```python
from build123d import *

# Parameters (mm, degrees)
F1_DEPTH = 12.7


with BuildPart() as f1:
    # F0 (on Right) → F1 (new body)
    with BuildSketch(Plane.YZ):
        with BuildLine():
            Line((-18.77171, -42.24451), (-18.77171, 60.838442))
            Line((-18.77171, 60.838442), (-29.627644, 60.838442))
            Line((-29.627644, 60.838442), (-29.627644, -38.221922))
            ThreePointArc((-29.627644, -38.221922), (-48.0446, -53.631362), (-69.885053, -43.64989))
            ThreePointArc((-69.885053, -43.64989), (-45.128132, -60.419661), (-19.449341, -45.098757))
            ThreePointArc((-19.449341, -45.098757), (-18.94344, -43.711302), (-18.77171, -42.24451))
        make_face()
    extrude(amount=F1_DEPTH)


solid = f1.part
```
For this review, take the finished solid that the model builds, in its own axes (mm). A direction names the side the tool comes from. Give positions to 0.01 mm unless a question says otherwise; leave off trailing zeros. Order: outer loops, then holes, each group sorted by start corner. A loop starts at its lowest first (then second) coordinate and runs counter-clockwise, first axis right, second up.
1) For faces 1 (the face through (12.7, -29, -8)), 2 (the face through (6, -29.628, 12)), list the 3-axis set-ups (+Z, -Z, +X, -X, +Y, -Y) from which the entire face can be reached by the end or side of a thin tool; tool diameter is ignored.
2) Take a section at A-A (x = 9.5). Give the boundary of the cut face in (y, z).
3) Wall thickness on line 1 (Y direction, x = 7.5, z = 51.5); line 2 (Y direction, x = 1.5, z = -51.5); line 3 (Z direction, x = 3.25, y = -40): over which ranges is each line inside the solid? List them lowest first.
4) Take a section at B-B (z = 19.5). Give the boundary of the cut face in (x, y), then the cut area to 3 significant figures.
5) Insertion check: pin 1 (4 mm diameter, centred on x = 8.5, z = 7, fed in from -Y); pin 2 (4 mm diameter, centred on x = 7.5, y = -30, fed in from -Z). Each pin has a flat end and moves straight along its axis. Give the tip position at first contact, or say it passes through.
6) Take a section at C-C (y = -43.5). Give the boundary of the cut face in (x, z), then the cut area to 3 significant figures.
Derived:
1. face 1: +Z, -Z, +X, +Y, -Y
1. face 2: +Z, +X, -X, -Y
2. outline: (-69.89, -43.65) arc R27.85 ccw to (-19.45, -45.1) arc R6.35 ccw to (-18.77, -42.24) - (-18.77, 60.84) - (-29.63, 60.84) - (-29.63, -38.22) arc R22.51 cw to start
3. line 1: y = -29.63 to -18.77
3. line 2: y = -64.77 to -61.03, -41.07 to -23.89
3. line 3: z = -60.09 to -50.93
4. outline: (0, -29.63) - (12.7, -29.63) - (12.7, -18.77) - (0, -18.77) - close
4. area: 138 mm2
5. pin 1: stops at y = -29.63
5. pin 2: stops at z = -57.55
6. outline: (0, -60.42) - (12.7, -60.42) - (12.7, -52.53) - (0, -52.53) - close
6. area: 100 mm2
